```python
from build123d import *

# Parameters (mm, degrees)
F1_DEPTH = 3.175
F2_DEPTH = 5.08
F3_T     = -1.6002


# Not quite as in the source:
# - a feature names something its author has since deleted; it is built from what else it names


with BuildPart() as f1:
    # F0 (on Top) → F1 (new body)
    with BuildSketch(Plane.XY):
        with BuildLine():
            Line((-6.9955831819, 8.5962191019), (-38.8090831819, 8.5962191019))
            Line((-38.8090831819, 8.5962191019), (-38.8090831819, 4.6274691019))
            Line((-38.8090831819, 4.6274691019), (-37.2342831819, 4.6274691019))
            ThreePointArc((-37.2342831819, 4.6274691019), (-34.8466831819, 7.0150691019), (-32.4590831819, 4.6274691019))
            Line((-32.4590831819, 4.6274691019), (-29.2840831819, 4.6274691019))
            ThreePointArc((-29.2840831819, 4.6274691019), (-26.8964831819, 7.0150691019), (-24.5088831819, 4.6274691019))
            Line((-24.5088831819, 4.6274691019), (-21.3338831819, 4.6274691019))
            ThreePointArc((-21.3338831819, 4.6274691019), (-18.9462831819, 7.0150691019), (-16.5586831819, 4.6274691019))
            Line((-16.5586831819, 4.6274691019), (-13.3836831819, 4.6274691019))
            ThreePointArc((-13.3836831819, 4.6274691019), (-10.9960831819, 7.0150691019), (-8.6084831819, 4.6274691019))
            Line((-8.6084831819, 4.6274691019), (-6.9955831819, 4.6274691019))
            Line((-6.9955831819, 4.6274691019), (-6.9955831819, 8.5962191019))
        make_face()
        with BuildLine():
            Line((-37.2342831819, 4.6274691019), (-38.8090831819, 4.6274691019))
            Line((-38.8090831819, 4.6274691019), (-38.8090831819, 0.6587191019))
            Line((-38.8090831819, 0.6587191019), (-6.9955831819, 0.6587191019))
            Line((-6.9955831819, 0.6587191019), (-6.9955831819, 4.6274691019))
            Line((-6.9955831819, 4.6274691019), (-8.6084831819, 4.6274691019))
            ThreePointArc((-8.6084831819, 4.6274691019), (-10.9960831819, 2.2398691019), (-13.3836831819, 4.6274691019))
            Line((-13.3836831819, 4.6274691019), (-16.5586831819, 4.6274691019))
            ThreePointArc((-16.5586831819, 4.6274691019), (-18.9462831819, 2.2398691019), (-21.3338831819, 4.6274691019))
            Line((-21.3338831819, 4.6274691019), (-24.5088831819, 4.6274691019))
            ThreePointArc((-24.5088831819, 4.6274691019), (-26.8964831819, 2.2398691019), (-29.2840831819, 4.6274691019))
            Line((-29.2840831819, 4.6274691019), (-32.4590831819, 4.6274691019))
            ThreePointArc((-32.4590831819, 4.6274691019), (-34.8466831819, 2.2398691019), (-37.2342831819, 4.6274691019))
        make_face()
        with BuildLine():
            Line((-37.2342831819, -3.3100308981), (-38.8090831819, -3.3100308981))
            Line((-38.8090831819, -3.3100308981), (-38.8090831819, -7.2787808981))
            Line((-38.8090831819, -7.2787808981), (-6.9955831819, -7.2787808981))
            Line((-6.9955831819, -7.2787808981), (-6.9955831819, -3.3100308981))
            Line((-6.9955831819, -3.3100308981), (-8.6084831819, -3.3100308981))
            ThreePointArc((-8.6084831819, -3.3100308981), (-10.9960831819, -5.6976308981), (-13.3836831819, -3.3100308981))
            Line((-13.3836831819, -3.3100308981), (-16.5586831819, -3.3100308981))
            ThreePointArc((-16.5586831819, -3.3100308981), (-18.9462831819, -5.6976308981), (-21.3338831819, -3.3100308981))
            Line((-21.3338831819, -3.3100308981), (-24.5088831819, -3.3100308981))
            ThreePointArc((-24.5088831819, -3.3100308981), (-26.8964831819, -5.6976308981), (-29.2840831819, -3.3100308981))
            Line((-29.2840831819, -3.3100308981), (-32.4590831819, -3.3100308981))
            ThreePointArc((-32.4590831819, -3.3100308981), (-34.8466831819, -5.6976308981), (-37.2342831819, -3.3100308981))
        make_face()
        with BuildLine():
            Line((-6.9955831819, 0.6587191019), (-38.8090831819, 0.6587191019))
            Line((-38.8090831819, 0.6587191019), (-38.8090831819, -3.3100308981))
            Line((-38.8090831819, -3.3100308981), (-37.2342831819, -3.3100308981))
            ThreePointArc((-37.2342831819, -3.3100308981), (-34.8466831819, -0.9224308981), (-32.4590831819, -3.3100308981))
            Line((-32.4590831819, -3.3100308981), (-29.2840831819, -3.3100308981))
            ThreePointArc((-29.2840831819, -3.3100308981), (-26.8964831819, -0.9224308981), (-24.5088831819, -3.3100308981))
            Line((-24.5088831819, -3.3100308981), (-21.3338831819, -3.3100308981))
            ThreePointArc((-21.3338831819, -3.3100308981), (-18.9462831819, -0.9224308981), (-16.5586831819, -3.3100308981))
            Line((-16.5586831819, -3.3100308981), (-13.3836831819, -3.3100308981))
            ThreePointArc((-13.3836831819, -3.3100308981), (-10.9960831819, -0.9224308981), (-8.6084831819, -3.3100308981))
            Line((-8.6084831819, -3.3100308981), (-6.9955831819, -3.3100308981))
            Line((-6.9955831819, -3.3100308981), (-6.9955831819, 0.6587191019))
        make_face()
    extrude(amount=F1_DEPTH)

    # F0 (on Top) → F2 (join)
    with BuildSketch(Plane.XY):
        with BuildLine():
            Line((-32.4590831819, 4.6274691019), (-37.2342831819, 4.6274691019))
            ThreePointArc((-37.2342831819, 4.6274691019), (-34.8466831819, 2.2398691019), (-32.4590831819, 4.6274691019))
        make_face()
        with BuildLine():
            ThreePointArc((-32.4590831819, 4.6274691019), (-34.8466831819, 7.0150691019), (-37.2342831819, 4.6274691019))
            Line((-37.2342831819, 4.6274691019), (-32.4590831819, 4.6274691019))
        make_face()
        with BuildLine():
            ThreePointArc((-32.4590831819, -3.3100308981), (-34.8466831819, -0.9224308981), (-37.2342831819, -3.3100308981))
            Line((-37.2342831819, -3.3100308981), (-32.4590831819, -3.3100308981))
        make_face()
        with BuildLine():
            Line((-32.4590831819, -3.3100308981), (-37.2342831819, -3.3100308981))
            ThreePointArc((-37.2342831819, -3.3100308981), (-34.8466831819, -5.6976308981), (-32.4590831819, -3.3100308981))
        make_face()
        with BuildLine():
            Line((-24.5088831819, -3.3100308981), (-29.2840831819, -3.3100308981))
            ThreePointArc((-29.2840831819, -3.3100308981), (-26.8964831819, -5.6976308981), (-24.5088831819, -3.3100308981))
        make_face()
        with BuildLine():
            ThreePointArc((-24.5088831819, -3.3100308981), (-26.8964831819, -0.9224308981), (-29.2840831819, -3.3100308981))
            Line((-29.2840831819, -3.3100308981), (-24.5088831819, -3.3100308981))
        make_face()
        with BuildLine():
            Line((-24.5088831819, 4.6274691019), (-29.2840831819, 4.6274691019))
            ThreePointArc((-29.2840831819, 4.6274691019), (-26.8964831819, 2.2398691019), (-24.5088831819, 4.6274691019))
        make_face()
        with BuildLine():
            ThreePointArc((-24.5088831819, 4.6274691019), (-26.8964831819, 7.0150691019), (-29.2840831819, 4.6274691019))
            Line((-29.2840831819, 4.6274691019), (-24.5088831819, 4.6274691019))
        make_face()
        with BuildLine():
            ThreePointArc((-21.3338831819, -3.3100308981), (-18.9462831819, -5.6976308981), (-16.5586831819, -3.3100308981))
            Line((-16.5586831819, -3.3100308981), (-21.3338831819, -3.3100308981))
        make_face()
        with BuildLine():
            Line((-21.3338831819, -3.3100308981), (-16.5586831819, -3.3100308981))
            ThreePointArc((-16.5586831819, -3.3100308981), (-18.9462831819, -0.9224308981), (-21.3338831819, -3.3100308981))
        make_face()
        with BuildLine():
            Line((-21.3338831819, 4.6274691019), (-16.5586831819, 4.6274691019))
            ThreePointArc((-16.5586831819, 4.6274691019), (-18.9462831819, 7.0150691019), (-21.3338831819, 4.6274691019))
        make_face()
        with BuildLine():
            ThreePointArc((-21.3338831819, 4.6274691019), (-18.9462831819, 2.2398691019), (-16.5586831819, 4.6274691019))
            Line((-16.5586831819, 4.6274691019), (-21.3338831819, 4.6274691019))
        make_face()
        with BuildLine():
            Line((-13.3836831819, -3.3100308981), (-8.6084831819, -3.3100308981))
            ThreePointArc((-8.6084831819, -3.3100308981), (-10.9960831819, -0.9224308981), (-13.3836831819, -3.3100308981))
        make_face()
        with BuildLine():
            ThreePointArc((-13.3836831819, -3.3100308981), (-10.9960831819, -5.6976308981), (-8.6084831819, -3.3100308981))
            Line((-8.6084831819, -3.3100308981), (-13.3836831819, -3.3100308981))
        make_face()
        with BuildLine():
            ThreePointArc((-13.3836831819, 4.6274691019), (-10.9960831819, 2.2398691019), (-8.6084831819, 4.6274691019))
            Line((-8.6084831819, 4.6274691019), (-13.3836831819, 4.6274691019))
        make_face()
        with BuildLine():
            Line((-13.3836831819, 4.6274691019), (-8.6084831819, 4.6274691019))
            ThreePointArc((-8.6084831819, 4.6274691019), (-10.9960831819, 7.0150691019), (-13.3836831819, 4.6274691019))
        make_face()
    extrude(amount=F2_DEPTH)

    # F3
    f3_openings = [f1.faces().sort_by_distance(p)[0] for p in [
        (-22.902333, 0.658719, 0),
    ]]
    offset(amount=F3_T, openings=f3_openings, kind=Kind.INTERSECTION)


solid = f1.part
```
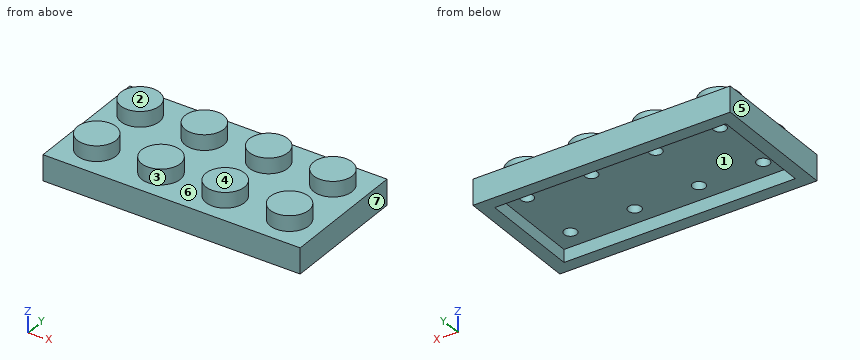
Can you work these out from the model? Positions are in its coordinate system, mm. Face numbers are marked on the shaded views. A direction names the side the tool comes from. Coordinates: 2 decimals unless noted, no trailing zeros. Loops run counter-clockwise (first coordinate to the right, second up) from the corner with the lowest first, then second, coordinate; pieces in that order, holes last.
Item 1: If we mould it in two halves opening along X, with no side actions, what happens to the marked faces 4, 5, 6 and 7? For each: released by +X, released by -X, zero draft, split by the parting line, or undercut.
Answers below:
face 4: zero draft
face 5: released by -X
face 6: undercut
face 7: released by +X
Item 2: Which directions (+Z, -Z, +X, -X, +Y, -Y) give clear straight access to the entire face, cutting with the end or side of a thin tool? Please do the marked faces 1, 2 and 3.
Answers below:
face 1: -Z
face 2: +Z, +X, -X, +Y, -Y
face 3: +Z
Item 3: Suppose I cut it at C-C (z = 3.9). Please give me the cut outline in (x, y), then the cut area to 3 significant figures.
Answers below:
outline: circle Ø4.78 at (-34.85, -3.31); circle Ø4.78 at (-34.85, 4.63); circle Ø4.78 at (-26.9, -3.31); circle Ø4.78 at (-26.9, 4.63); circle Ø4.78 at (-18.95, -3.31); circle Ø4.78 at (-18.95, 4.63); circle Ø4.78 at (-11, -3.31); circle Ø4.78 at (-11, 4.63)
area: 143 mm2
Item 4: I'm going to push flat-ended pins straight in: pin 1 (1.7 mm diameter, centred on x = -35, y = -3, fed in from -Z); pin 2 (8 mm diameter, centred on x = -20, y = 0.5, fed in from +Z); pin 3 (0.5 mm diameter, centred on x = -19, y = 5, fed in from -Z). Where does each tip first touch, or does it pass through?
Answers below:
pin 1: stops at z = 1.57
pin 2: stops at z = 5.08
pin 3: stops at z = 3.48
Item 5: Suppose I cut it at A-A (y = 1.75). Please give me the cut outline in (x, z) (3 decimals), then the cut area to 3 significant figures.
Answers below:
outline: (-38.809, 0) - (-37.209, 0) - (-37.209, 1.575) - (-8.596, 1.575) - (-8.596, 0) - (-6.996, 0) - (-6.996, 3.175) - (-38.809, 3.175) - close
area: 55.9 mm2
Item 6: Please list where these lines run through material, in increasing order: L1, parallel to Y at x = -16.5, z = 0.85; L2, parallel to X at y = 4.75, z = 4.2; L3, parallel to X at y = -4.75, z = 4.3.
Answers below:
L1: y = -7.28 to -5.68, 7 to 8.6
L2: x = -37.23 to -32.46, -29.28 to -24.51, -21.33 to -16.56, -13.38 to -8.61
L3: x = -36.75 to -32.94, -28.8 to -24.99, -20.85 to -17.04, -12.9 to -9.09
Item 7: Suppose I cut it at B-B (x = -31). Please give me the cut outline in (y, z) (3 decimals).
Answers below:
outline: (-7.279, 0) - (-5.679, 0) - (-5.679, 1.575) - (6.996, 1.575) - (6.996, 0) - (8.596, 0) - (8.596, 3.175) - (-7.279, 3.175) - close
Item 8: Suppose I cut it at D-D (y = -5). Please give me the cut outline in (x, z) (3 decimals), then the cut area to 3 significant figures.
Answers below:
outline: (-38.809, 0) - (-37.209, 0) - (-37.209, 1.575) - (-8.596, 1.575) - (-8.596, 0) - (-6.996, 0) - (-6.996, 3.175) - (-9.309, 3.175) - (-9.309, 5.08) - (-12.683, 5.08) - (-12.683, 3.175) - (-17.26, 3.175) - (-17.26, 5.08) - (-20.633, 5.08) - (-20.633, 3.175) - (-25.21, 3.175) - (-25.21, 5.08) - (-28.583, 5.08) - (-28.583, 3.175) - (-33.16, 3.175) - (-33.16, 5.08) - (-36.533, 5.08) - (-36.533, 3.175) - (-38.809, 3.175) - close
area: 81.7 mm2
